Work out the finished part from the listing and answer in its coordinate system (mm). Face numbers are marked on the shaded views. A direction names the side the tool comes from. Coordinates: 2 decimals unless noted, no trailing zeros. Loops run counter-clockwise (first coordinate to the right, second up) from the corner with the lowest first, then second, coordinate; pieces in that order, holes last. Notation, with made-up numbers: M 59,-5 L 112,-5 A25 ccw 112,26 Z; hole C 56,87.5 d9. An arc over 180 degrees is marked long. Write each question's results on one line, items separated by ' | '.
```python
from build123d import *

# Parameters (mm, degrees)
F0_R     = 40.64
F0_R_2   = 2.54
F1_DEPTH = 6.35
F3_R     = 35.814
F4_DEPTH = 2.413
F5_DEPTH = 8.764


with BuildPart() as f1:
    # F0 (on Top) → F1 (new body)
    with BuildSketch(Plane.XY):
        Circle(F0_R)
        Circle(F0_R_2, mode=Mode.SUBTRACT)
    extrude(amount=F1_DEPTH)

    # F3 (on face) → F4 (join)
    with BuildSketch(Plane(origin=(0, 0, 0), x_dir=(1, 0, 0), z_dir=(0, 0, -1))):
        Circle(F3_R)
    extrude(amount=F4_DEPTH)

    # F2 (on face) → F5 (cut, through all)
    with BuildSketch(Plane.XY.offset(6.35)):
        with BuildLine():
            Line((-26.1582, 17.994751), (26.1582, 17.994751))
            ThreePointArc((26.1582, 17.994751), (24.117564, 20.649591), (21.808676, 23.074751))
            Line((21.808676, 23.074751), (-21.808676, 23.074751))
            ThreePointArc((-21.808676, 23.074751), (-24.117564, 20.649591), (-26.1582, 17.994751))
        make_face()
        with BuildLine():
            Line((0, 2.54), (-31.648237, 2.54))
            ThreePointArc((-31.648237, 2.54), (-31.75, 0), (-31.648237, -2.54))
            Line((-31.648237, -2.54), (31.648237, -2.54))
            ThreePointArc((31.648237, -2.54), (31.75, 0), (31.648237, 2.54))
            Line((31.648237, 2.54), (0, 2.54))
        make_face()
        with BuildLine():
            ThreePointArc((-29.004684, 12.914751), (-29.994159, 10.412152), (-30.768152, 7.834751))
            Line((-30.768152, 7.834751), (30.768152, 7.834751))
            ThreePointArc((30.768152, 7.834751), (29.994159, 10.412152), (29.004684, 12.914751))
            Line((29.004684, 12.914751), (-29.004684, 12.914751))
        make_face()
        with BuildLine():
            Line((-14.675575, 28.154751), (14.675575, 28.154751))
            ThreePointArc((14.675575, 28.154751), (0, 31.75), (-14.675575, 28.154751))
        make_face()
        with BuildLine():
            Line((30.822039, -7.62), (-30.822039, -7.62))
            ThreePointArc((-30.822039, -7.62), (-30.068172, -10.196446), (-29.099356, -12.7))
            Line((-29.099356, -12.7), (29.099356, -12.7))
            ThreePointArc((29.099356, -12.7), (30.068172, -10.196446), (30.822039, -7.62))
        make_face()
        with BuildLine():
            Line((26.448526, -17.565249), (-26.448526, -17.565249))
            ThreePointArc((-26.448526, -17.565249), (-24.483538, -20.214323), (-22.25433, -22.645249))
            Line((-22.25433, -22.645249), (22.25433, -22.645249))
            ThreePointArc((22.25433, -22.645249), (24.483538, -20.214323), (26.448526, -17.565249))
        make_face()
        with BuildLine():
            Line((15.471686, -27.725249), (-15.471686, -27.725249))
            ThreePointArc((-15.471686, -27.725249), (0, -31.75), (15.471686, -27.725249))
        make_face()
    extrude(amount=-F5_DEPTH, mode=Mode.SUBTRACT)


solid = f1.part
```
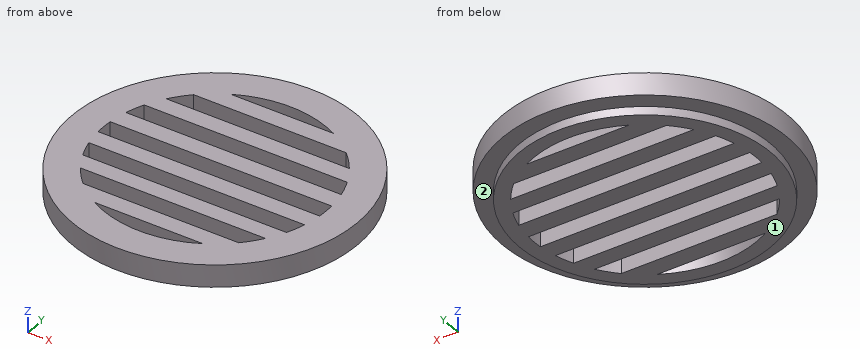
1) Find section A-A, the plane y = 0. Give the vertices of the cut face in (x, z).
Check result:
outline: M -40.64,0 L -35.81,0 L -35.81,-2.41 L -31.75,-2.41 L -31.75,6.35 L -40.64,6.35 Z; M 31.75,-2.41 L 35.81,-2.41 L 35.81,0 L 40.64,0 L 40.64,6.35 L 31.75,6.35 Z
2) Find section C-C, the plane z = -1.25. Give the vertices of the cut face in (x, y).
Check result:
outline: C 0,0 d71.63; hole M -31.65,-2.54 L 31.65,-2.54 A31.75 ccw 31.65,2.54 L -31.65,2.54 A31.75 ccw Z; hole M -30.82,-7.62 A31.75 ccw -29.1,-12.7 L 29.1,-12.7 A31.75 ccw 30.82,-7.62 Z; hole M -30.77,7.83 L 30.77,7.83 A31.75 ccw 29,12.91 L -29,12.91 A31.75 ccw Z; hole M -26.45,-17.57 A31.75 ccw -22.25,-22.65 L 22.25,-22.65 A31.75 ccw 26.45,-17.57 Z; hole M -26.16,17.99 L 26.16,17.99 A31.75 ccw 21.81,23.07 L -21.81,23.07 A31.75 ccw Z; hole M -15.47,-27.73 A31.75 ccw 15.47,-27.73 Z; hole M -14.68,28.15 L 14.68,28.15 A31.75 ccw Z
3) Straight lines are drawn through the part: probe 1 along Y at (x, z) = (27, 4.25); probe 2 along Y at (x, z) = (20.5, 6.25); probe 3 along Y at (x, z) = (-25, 5). For each, find the intervals that lie inside material, in ascending order. Write a range as [from, to].
Check result:
probe 1: [-30.37, -12.7], [-7.62, -2.54], [2.54, 7.83], [12.91, 30.37] | probe 2: [-35.09, -22.65], [-17.57, -12.7], [-7.62, -2.54], [2.54, 7.83], [12.91, 17.99], [23.07, 35.09] | probe 3: [-32.04, -19.57], [-17.57, -12.7], [-7.62, -2.54], [2.54, 7.83], [12.91, 17.99], [19.57, 32.04]
4) Which of the six approach directions +Z, -Z, +X, -X, +Y, -Y give full straight-line access (tool end or side, diameter ignored) to the marked faces 1 and 2?
Check result:
face 1: -Z, +X, -X, +Y, -Y | face 2: -Z
5) Given pin 1 Ø1.5 at (x, z) = (-12, 1.5) entering from -Y; pin 2 Ø1 at (x, z) = (-32.5, 5.5) entering from -Y; pin 3 Ø2.5 at (x, z) = (-13, 2.5) entering from +Y, each flat-ended and moving along its own axis, determine where each tip first touches the part or whether it passes through.
Check result:
pin 1: y = -39.05 | pin 2: y = -25.05 | pin 3: y = 38.9
6) Find section D-D, the plane x = 34.5. Give the vertices of the cut face in (y, z).
Check result:
outline: M -21.48,0 L -9.61,0 L -9.61,-2.41 L 9.61,-2.41 L 9.61,0 L 21.48,0 L 21.48,6.35 L -21.48,6.35 Z
7) Find section B-B, the plane x = 17. Give the vertices of the cut face in (y, z), and give its area (3 significant figures).
Check result:
outline: M -36.91,0 L -31.52,0 L -31.52,-2.41 L -22.65,-2.41 L -22.65,6.35 L -36.91,6.35 Z; M -17.57,-2.41 L -12.7,-2.41 L -12.7,6.35 L -17.57,6.35 Z; M -7.62,-2.41 L -2.54,-2.41 L -2.54,6.35 L -7.62,6.35 Z; M 2.54,-2.41 L 7.83,-2.41 L 7.83,6.35 L 2.54,6.35 Z; M 12.91,-2.41 L 17.99,-2.41 L 17.99,6.35 L 12.91,6.35 Z; M 23.07,-2.41 L 31.52,-2.41 L 31.52,0 L 36.91,0 L 36.91,6.35 L 23.07,6.35 Z | area: 398 mm^2
